```python
from build123d import *

# Parameters (mm, degrees)
SKETCH_1_R          = 24.5
EXTRUDE_3_DEPTH     = 2
SKETCH_3_R          = 1.9
CUT_EXTRUDE_1_DEPTH = 3
SKETCH_4_R          = 18.026762753
EXTRUDE_4_DEPTH     = 30
SKETCH_5_R          = 42.5
EXTRUDE_6_DEPTH     = 2.5
SKETCH_6_R          = 25
SKETCH_6_R_2        = 23.5
EXTRUDE_7_DEPTH     = 2


with BuildPart() as part:
    # 스케치1 → 보스-돌출3 (new body)
    with BuildSketch(Plane.XY):
        with Locations((4.325882057, 117.219920175)):
            Circle(SKETCH_1_R)
    extrude(amount=EXTRUDE_3_DEPTH)

    # 스케치3 → 컷-돌출1 (cut)
    with BuildSketch(Plane.XY.offset(2)):
        with Locations((1.179008368, 95.896439246)):
            Circle(SKETCH_3_R)
        with Locations((22.395703109, 124.906718796)):
            Circle(SKETCH_3_R)
        with Locations((-13.882118572, 128.141421182)):
            Circle(SKETCH_3_R)
    extrude(amount=-CUT_EXTRUDE_1_DEPTH, mode=Mode.SUBTRACT)

    # 스케치4 → 보스-돌출4 (add)
    with BuildSketch(Plane.XY.offset(2)):
        with Locations((3.749565529, 116.53268792)):
            Circle(SKETCH_4_R)
    extrude(amount=EXTRUDE_4_DEPTH)

    # 스케치5 → 보스-돌출6 (add)
    with BuildSketch(Plane.XY.offset(32)):
        with Locations((3.749565529, 116.53268792)):
            Circle(SKETCH_5_R)
    extrude(amount=EXTRUDE_6_DEPTH)

    # 스케치6 → 보스-돌출7 (add)
    with BuildSketch(Plane.XY.offset(34.5)):
        with Locations((3.749565529, 116.53268792)):
            Circle(SKETCH_6_R)
        with Locations((3.749565529, 116.53268792)):
            Circle(SKETCH_6_R_2, mode=Mode.SUBTRACT)
    extrude(amount=EXTRUDE_7_DEPTH)


solid = part.part
```
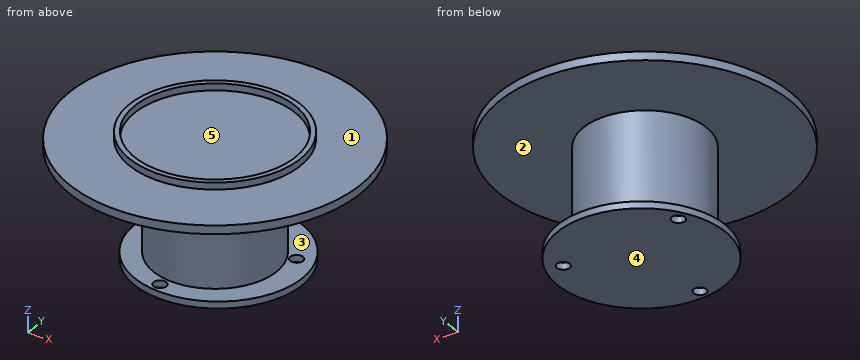
Verification items for the finished model (mm, model axes). Face numbers are marked on the shaded views. A direction names the side the tool comes from. Coordinates: 2 decimals unless noted, no trailing zeros. Write each loop counter-clockwise with the first axis right and the second up, starting at its lowest first coordinate (ties: lowest second). Pieces come first, ordered by that corner, then holes. Notation, with made-up numbers: (57, 10) - (77, 10) arc R28 ccw to (77, 45) - close; hole circle Ø3 at (5.5, -9.75). An arc over 180 degrees is marked (long way). One line per question, with ' | ' between items. Start each with the question number.
1. Section check D-D (x = 30.5). Enter the section's corners in (y, z).
2. Access from +Z, -Z, +X, -X, +Y, -Y to the whole of each face (thin tool, end or side, straight path). Record for the marked faces 1 and 2.
3. Section check B-B (x = 11). Enter the section's corners in (y, z).
4. Draft check along Z on the marked faces 3, 4 and 5. Enter one of: released by +Z, released by -Z, zero draft, split by the parting line, or undercut.
5. Gauge pin test, flat ends, axial feed: P1, Ø10, axis at x = -4, z = 20.5, coming from the +Y side; P2, Ø5, axis at x = -13.88, y = 128.14, coming from the +Z side; P3, Ø5, axis at x = 21.5, z = 5.5, coming from the +Y side; P4, Ø4, axis at x = -19.5, y = 86, coming from the -Z side. Record the tip position at first contact, or that the pin passes through.
6. Section check C-C (z = 4.5). Enter the section's corners in (x, y), plus the area to 3 significant figures.
7. Material ranges on line 1 along Z through (x, y) = (-13.5, 133); line 2 along Z through (x, y) = (9, 95); line 3 along Z through (x, y) = (38.5, 134), recorded low to high.
8. Section check A-A (y = 101). Enter the section's corners in (x, z).
Computed values:
1) outline: (83.51, 32) - (149.56, 32) - (149.56, 34.5) - (83.51, 34.5) - close
2) face 1: +Z | face 2: none
3) outline: (74.66, 32) - (100.03, 32) - (100.03, 2) - (93.65, 2) - (93.65, 0) - (140.79, 0) - (140.79, 2) - (133.04, 2) - (133.04, 32) - (158.41, 32) - (158.41, 34.5) - (140.46, 34.5) - (140.46, 36.5) - (138.89, 36.5) - (138.89, 34.5) - (94.18, 34.5) - (94.18, 36.5) - (92.61, 36.5) - (92.61, 34.5) - (74.66, 34.5) - close
4) face 3: undercut | face 4: released by -Z | face 5: released by +Z
5) P1: y = 134.35 | P2: z = 36.5 | P3: y = 126.14 | P4: z = 32
6) outline: circle Ø36.05 at (3.75, 116.53) | area: 1,020 mm²
7) line 1: 0 to 2, 32 to 36.5 | line 2: 0 to 2, 32 to 34.5 | line 3: 32 to 34.5
8) outline: (-35.81, 32) - (-5.4, 32) - (-5.4, 2) - (-14.04, 2) - (-14.04, 0) - (22.69, 0) - (22.69, 2) - (12.9, 2) - (12.9, 32) - (43.31, 32) - (43.31, 34.5) - (23.34, 34.5) - (23.34, 36.5) - (21.38, 36.5) - (21.38, 34.5) - (-13.89, 34.5) - (-13.89, 36.5) - (-15.84, 36.5) - (-15.84, 34.5) - (-35.81, 34.5) - close
